Autodesk Inventor part; units mm, degrees
ref_plane "YZ Plane" through (0, 0, 0) normal (1, 0, 0) x (0, 1, 0)
ref_plane "XZ Plane" through (0, 0, 0) normal (0, 1, 0) x (-1, 0, 0)
ref_plane "XY Plane" through (0, 0, 0) normal (0, 0, 1) x (1, 0, 0)
sketch "Boceto1" plane through (0, 0, 0) normal (0, 0, 1) x (1, 0, 0)
  line L0 (0, 50) -> (0, -50) construction
  line L1 (-50, 0) -> (50, 0) construction
  line L2 (-50, -52) -> (50, -52) construction
  circle A0 centre (0, -52) radius 10
  circle A1 centre (0, 0) radius 6.5
  arc A2 (13.4711, 6.5977) -> (-15, 0) centre (0, 0) ccw
  arc A3 (-15, -13.2288) -> (17.3205, -10) centre (0, 0) ccw
  line L3 (17.3205, -10) -> (25, -10)
  line L4 (40, -56) -> (65, -56)
  line L5 (65, -56) -> (65, -66)
  line L6 (65, -66) -> (40, -66)
  line L7 (-15, 0) -> (-15, -66)
  line L8 (65, 25.2383) -> (65, -76.5705) construction
  line L9 (40, -66) -> (-15, -66)
  line L10 (40, -41) -> (65, -41)
  arc A4 (40, -41) -> (40, -56) centre (40, -48.5) ccw
  line L11 (65, -41) -> (65, -31)
  line L12 (25, 28.6395) -> (25, -70.532) construction
  arc A5 (25, -10) -> (65, -31) centre (75.7977, 38.1622) ccw
  arc A6 (13.4711, 6.5977) -> (25, -10) centre (73.5302, 36.0124) ccw
  point P0 (0, 0)
  point P1 (17.3859, -10)
  point P2 (65, -61)
  point P3 (40, -61)
  point P4 (52.5, -41)
  dimension "d0" = 100
  dimension "d1" = 100
  dimension "d2" = 52
  dimension "d3" = 100
  dimension "d4" = 20
  dimension "d5" = 13
  dimension "d6" = 15
  dimension "d7" = 20
  dimension "d8" = 10
  dimension "d9" = 56
  dimension "d10" = 10
  dimension "d11" = 25
  dimension "d12" = 80
  dimension "d14" = 15
  dimension "d15" = 7.5
  dimension "d16" = 7.5
  dimension "d17" = 25
  dimension "d18" = 10
  dimension "d19" = 40
  dimension "d20" = 25
  dimension "d21" = 80
  dimension "d22" = 70
  dimension "d23" = 7.6141
extrude "Extrusión1" add sketch "Boceto1" along normal mid plane 15 contours A6 L3 A3 L7 A2
extrude "Extrusión2" add sketch "Boceto1" along normal mid plane 30 contours A5 L11 L10 A4 L4 L5 L6 L9 L7 A3 L3
fillet "Empalme1" radius 14 1 edges at (-15, -66, 0)
sketch "Boceto2" plane through (65, -66, -15) normal (0, -1, 0) x (1, 0, 0)
  line L0 (0, 0) -> (0, 30)
  line L1 (0, 22.5) -> (-40, 22.5)
  line L2 (-40, 22.5) -> (-40, 7.5)
  line L3 (-40, 7.5) -> (0, 7.5)
  line L4 (0, 7.5) -> (0, 22.5)
  line L5 (38.7229, 15) -> (-93.8867, 15) construction
  point P0 (-65, 15)
  point P1 (0, 7.5)
  dimension "d29" = 40
  dimension "d30" = 15
  dimension "d31" = 15
  dimension "d32" = 132.6097
  dimension "d33" = 38.7229
extrude "Extrusión3" cut sketch "Boceto2" against normal blind 50
properties part number "ensayo 8" material "Acero inoxidable"
Geometry check sheet. Reference: the model listing, model coordinates, mm. A direction names the side the tool comes from. Coordinates: 2 decimals unless noted, no trailing zeros. Write each loop counter-clockwise with the first axis right and the second up, starting at its lowest first coordinate (ties: lowest second). Pieces come first, ordered by that corner, then holes. Notation, with made-up numbers: (52, 85) -> (99, 85) arc R24 cw to (99, 103) -> close; hole circle Ø3 at (-24, 76.5). An arc over 180 degrees is marked (long way). Use CSV: the item, a comma, the result in double quotes. Start each with the question number.
Item 1: Mould release check, pull along Z, two halves, no side actions. Record for faces 1 (the flat face through (5, -6, 7.5)), 2 (the flat face through (25, -41, 0)), 3 (the flat face through (52, -41, -11)): released by +Z, released by -Z, zero draft, split by the parting line, or undercut.
Item 2: Cross-section at D-D, the plane y = -39. Record the cut outline in (x, z), plus the area to 3 significant figures.
Item 3: Depth check by flat-ended pin: pin 1 Ø8 at (x, z) = (22, -10) entering from +Y; pin 2 Ø8 at (x, z) = (48, -10.5) entering from +Y; pin 3 Ø6 at (x, z) = (52, 12.5) entering from +Y. Enter the tip coordinate at first touch or a pass-through.
Item 4: Cross-section at B-B, the plane x = 0. Record the cut outline in (y, z).
Item 5: Thickness scan on line 1 (Y direction, x = 0, z = -2.25); line 2 (Z direction, x = 28.5, y = -53.5); line 3 (Y direction, x = -5, z = 5.75). Record the ranges inside material, lowest first.
Item 6: Cross-section at C-C, the plane z = 3.25. Record the cut outline in (x, y), plus the area to 3 significant figures.
Item 7: Set-up check for faces 4 (the cylindrical face through (2.252, -19.873, -11.302)), 5 (the flat face through (28, -16, 0)), 6 (the flat face through (21, -10, -11)), 7 (the flat face through (52, -56, 11)): record each of +Z, -Z, +X, -X, +Y, -Y from which the full face is reachable in a straight line by a thin tool's end or side.
Item 8: Cross-section at A-A, the plane y = -48.5. Record the cut outline in (x, z).
Answers:
1,face 1,"released by +Z"
1,face 2,"undercut"
1,face 3,"zero draft"
2,outline,"(-15, -15) -> (65, -15) -> (65, -7.5) -> (25, -7.5) -> (25, 7.5) -> (65, 7.5) -> (65, 15) -> (-15, 15) -> close"
2,area,"1,800 mm^2"
3,pin 1,"y = -2.53"
3,pin 2,"y = -24.2"
3,pin 3,"y = -26.51"
4,outline,"(-66, -15) -> (-62, -15) -> (-62, 15) -> (-66, 15) -> close; (-42, -15) -> (-20, -15) -> (-20, -7.5) -> (-6.5, -7.5) -> (-6.5, 7.5) -> (-20, 7.5) -> (-20, 15) -> (-42, 15) -> close; (6.5, -7.5) -> (15, -7.5) -> (15, 7.5) -> (6.5, 7.5) -> close"
5,line 1,"-66 to -62, -42 to -6.5, 6.5 to 15"
5,line 2,"-15 to -7.5, 7.5 to 15"
5,line 3,"-65.42 to -60.66, -43.34 to -4.15, 4.15 to 14.14"
6,outline,"(-15, -52) arc R14 ccw to (-1, -66) -> (25, -66) -> (25, -16) -> (31.45, -16) arc R70 cw to (25, -10) arc R66.88 cw to (13.47, 6.6) arc R15 ccw to (-15, 0) -> close; hole circle Ø20 at (0, -52); hole circle Ø13 at (0, 0)"
6,area,"2,490 mm^2"
7,face 4,"-Z, +Y"
7,face 5,"+X, -Y"
7,face 6,"-Z, +X, -X, +Y"
7,face 7,"+Z, -Z, +X"
8,outline,"(-15, -15) -> (-9.37, -15) -> (-9.37, 15) -> (-15, 15) -> close; (9.37, -15) -> (32.5, -15) -> (32.5, -7.5) -> (25, -7.5) -> (25, 7.5) -> (32.5, 7.5) -> (32.5, 15) -> (9.37, 15) -> close"
